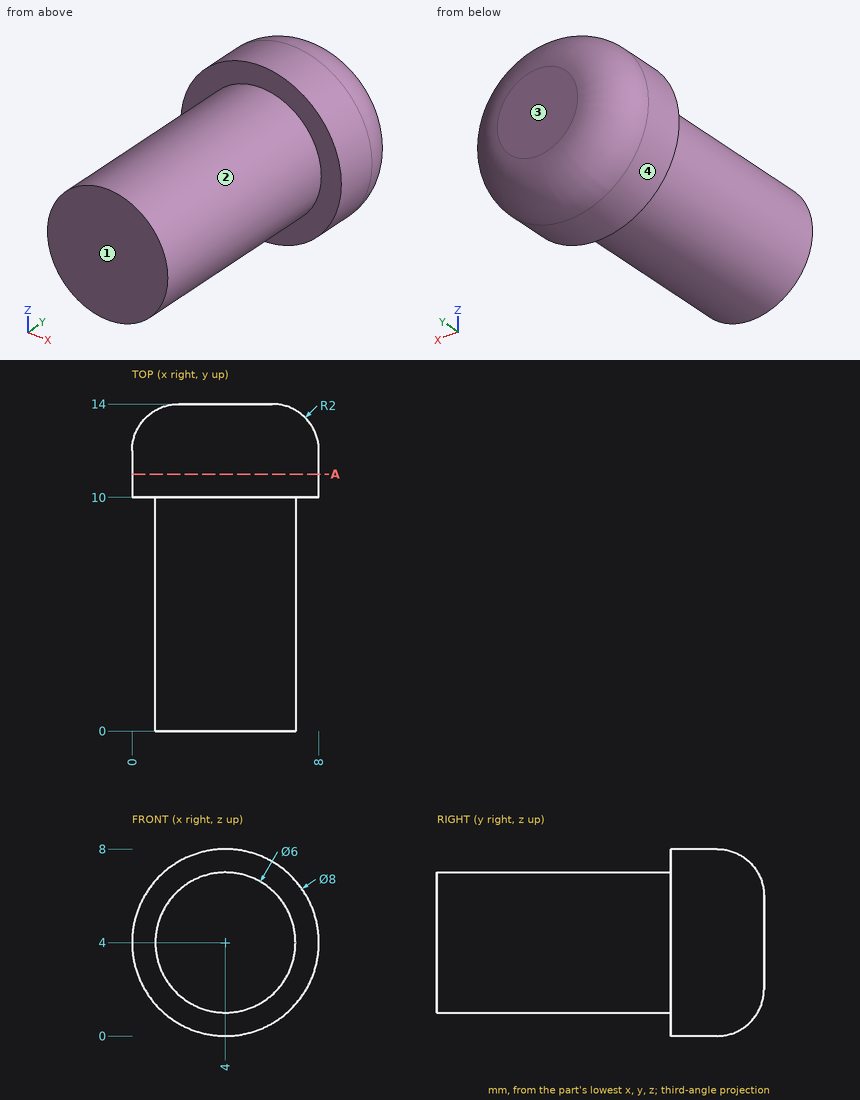
Study the drawing (mm; zero at the part's minimum x, y, z) and answer. A direction names the side the tool comes from. Coordinates: 2 decimals unless noted, no trailing zeros. Write each loop counter-clockwise with the first axis right and the second up, starting at its lowest first coordinate (ties: lowest second). Pieces come first, ordered by that corner, then holes. Notation, with made-up numbers: (66, -8) - (78, -8) arc R14 cw to (78, -3) - close; hole circle Ø1 at (-28.75, 53.5). An arc over 180 degrees is marked (long way). One line per item, written item: value.
1) A tool of negligible diameter and unlimited length cuts with its end or side. For the marked faces 1 and 2, from which of +Z, -Z, +X, -X, +Y, -Y can it reach the whole face along a straight path? Write none if from no direction.
Geometry check:
face 1: +Z, -Z, +X, -X, -Y
face 2: -Y
2) For a pull along Z with two mould halves and no side action, classify the marked faces 3 and 4 as pulls with the +Z half, pulls with the -Z half, needs draft (parallel to the pull), parting line crosses it, or undercut.
Geometry check:
face 3: needs draft
face 4: parting line crosses it
3) Consider line 1 along Z through (x, y) = (2.25, 7); line 2 along Z through (x, y) = (2.5, 3.75); line 3 along Y through (x, z) = (6.75, 3). Determine where each line is inside the solid, lowest interval first. Write a range as from..to.
Geometry check:
line 1: z = 1.56..6.44
line 2: z = 1.4..6.6
line 3: y = 0..13.77
4) Find section A-A (y = 11). Give the vertices of the cut face in (x, z).
Geometry check:
outline: circle Ø8 at (4, 4)
5) Each of these flat-tipped pins is pushed along its axis until it touches: pin 1 Ø3 at (x, y) = (3, 3) entering from +Z; pin 2 Ø1.5 at (y, z) = (6, 6) entering from -X; pin 3 Ø1.5 at (y, z) = (10, 2.5) entering from -X. Where does it stop, or does it pass through?
Geometry check:
pin 1: stops at z = 7
pin 2: stops at x = 1.27
pin 3: stops at x = 0.07
